```python
from build123d import *

# Parameters (mm, degrees)
F0_R     = 4.5
F1_DEPTH = 3.175
F0_R_2   = 2.25
F2_DEPTH = 1.5875
F3_DEPTH = 13.97
F4_W     = 8.5852
F4_H     = 8.4761770735
F5_DEPTH = 25.4
F6_R     = 3.81


with BuildPart() as f1:
    # F0 (on Top) → F1 (new body)
    with BuildSketch(Plane.XY):
        with BuildLine():
            Line((6.5, -8.5852), (6.5, 0))
            ThreePointArc((6.5, 0), (0, -6.5), (-6.5, 0))
            Line((-6.5, 0), (-6.5, -8.5852))
            Line((-6.5, -8.5852), (6.5, -8.5852))
        make_face()
        with BuildLine():
            ThreePointArc((-6.5, 0), (0, -6.5), (6.5, 0))
            ThreePointArc((6.5, 0), (0, 6.5), (-6.5, 0))
        make_face()
        Circle(F0_R, mode=Mode.SUBTRACT)
    extrude(amount=F1_DEPTH)

    # F0 (on Top) → F2 (join)
    with BuildSketch(Plane.XY):
        Circle(F0_R)
        Circle(F0_R_2, mode=Mode.SUBTRACT)
    extrude(amount=F2_DEPTH)

    # F0 (on Top) → F3 (join)
    with BuildSketch(Plane.XY):
        with BuildLine():
            Line((6.5, -24.3332), (6.5, -8.5852))
            Line((6.5, -8.5852), (-6.5, -8.5852))
            Line((-6.5, -8.5852), (-6.5, -24.3332))
            ThreePointArc((-6.5, -24.3332), (-5.3840768363, -27.0272768363), (-2.69, -28.1432))
            Line((-2.69, -28.1432), (2.69, -28.1432))
            ThreePointArc((2.69, -28.1432), (5.3840768363, -27.0272768363), (6.5, -24.3332))
        make_face()
    extrude(amount=F3_DEPTH)

    # F4 (on face) → F5 (cut)
    with BuildSketch(Plane.YZ.offset(6.5)):
        with BuildLine():
            ThreePointArc((-12.6179837447, 3.175), (-9.7820030962, 4.5000062934), (-8.6270184297, 7.4093770735))
            ThreePointArc((-8.6270184297, 7.4093770735), (-9.8694128853, 10.408782618), (-12.8688184297, 11.6511770735))
            Line((-12.8688184297, 11.6511770735), (-12.8688184297, 3.175))
            Line((-12.8688184297, 3.175), (-12.6179837447, 3.175))
        make_face()
        with BuildLine():
            Line((-12.8688184297, 3.175), (-12.8688184297, 11.6511770735))
            ThreePointArc((-12.8688184297, 11.6511770735), (-17.108762292, 7.2839048265), (-12.6179837447, 3.175))
            Line((-12.6179837447, 3.175), (-12.8688184297, 3.175))
        make_face()
        with Locations((-4.2926, 7.4130885368)):
            Rectangle(F4_W, F4_H)
        with BuildLine():
            ThreePointArc((-12.8688184297, 11.6511770735), (-9.8694128853, 10.408782618), (-8.6270184297, 7.4093770735))
            ThreePointArc((-8.6270184297, 7.4093770735), (-9.7820030962, 4.5000062934), (-12.6179837447, 3.175))
            Line((-12.6179837447, 3.175), (-8.5852, 3.175))
            Line((-8.5852, 3.175), (-8.5852, 11.6511770735))
            Line((-8.5852, 11.6511770735), (-12.8688184297, 11.6511770735))
        make_face()
    extrude(amount=-F5_DEPTH, mode=Mode.SUBTRACT)

    # F6
    f6_edges = [f1.edges().sort_by_distance(p)[0] for p in [
        (6.5, -8.5852, 12.810589),
        (-6.5, -8.5852, 12.810589),
    ]]
    fillet(f6_edges, radius=F6_R)


solid = f1.part
```
The model under review builds one solid part; all positions refer to its coordinate system, in mm. A direction names the side the tool comes from. Give positions to 0.01 mm unless a question says otherwise; leave off trailing zeros. Loops run counter-clockwise (first coordinate to the right, second up) from the corner with the lowest first, then second, coordinate; pieces in that order, holes last. Notation, with made-up numbers: (-24, 67.25) - (-2, 67.25) arc R19 cw to (-2, 88.25) - close; hole circle Ø6 at (26.25, 62.5). An arc over 180 degrees is marked (long way). Answer as a JSON object with one key per item and string values.
Q1. Mouldability with a two-part tool opening along Y and no side actions: class faces 1 (the cylindrical face through (-0.59, 4.46, 2.37)), 2 (the flat face through (0, -8.585, 13)), 3 (the cylindrical face through (5.35, -27.06, 6.89)) as +Y half, -Y half, draft (parallel to the pull), parting line (faces both ways), or undercut.
Worked out:
{"face 1": "undercut", "face 2": "+Y half", "face 3": "-Y half"}
Q2. Add section B-B on y = -9.5. State the section outline as (x, z) points (3 decimals), plus the area to 3 significant figures.
Worked out:
{"outline": "(-6.5, 0) - (6.5, 0) - (6.5, 3.175) - (-6.5, 3.175) - close; (-5.167, 11.651) - (5.167, 11.651) - (5.167, 13.97) - (-5.167, 13.97) - close", "area": "65.2 mm^2"}
Q3. For faces 4 (the flat face through (0, -11, 11.651)), 5 (the cylindrical face through (5.41, -9.73, 12.83)), 6 (the cylindrical face through (-5.41, -9.73, 12.83)), 7 (the flat face through (2, -2, 1.588)), list the 3-axis set-ups (+Z, -Z, +X, -X, +Y, -Y) from which the entire face can be reached by the end or side of a thin tool; tool diameter is ignored.
Worked out:
{"face 4": "+X, -X, +Y", "face 5": "+Z, +X, +Y", "face 6": "+Z, -X, +Y", "face 7": "+Z"}
Q4. Add section C-C on z = 12.25. State the section outline as (x, y) points, plus the area to 3 significant figures.
Worked out:
{"outline": "(-6.5, -24.33) arc R3.81 ccw to (-2.69, -28.14) - (2.69, -28.14) arc R3.81 ccw to (6.5, -24.33) - (6.5, -12.4) arc R3.81 ccw to (2.69, -8.59) - (-2.69, -8.59) arc R3.81 ccw to (-6.5, -12.4) - close", "area": "242 mm^2"}
Q5. To check wall thickness, follow line 1 along Y through (x, z) = (0, 0.75); line 2 along Z through (x, y) = (0.75, -9.5) (3 decimals); line 3 along Y through (x, z) = (-2.25, 12.75). State the ranges of each line that lie inside material, in increasing order.
Worked out:
{"line 1": "y = -28.14 to -2.25, 2.25 to 6.5", "line 2": "z = 0 to 3.175, 11.651 to 13.97", "line 3": "y = -28.14 to -8.59"}
Q6. Add section D-D on y = -3.5. State the section outline as (x, z) points (1 decimal), plus the area to 3 significant figures.
Worked out:
{"outline": "(-6.5, 0) - (6.5, 0) - (6.5, 3.2) - (2.8, 3.2) - (2.8, 1.6) - (-2.8, 1.6) - (-2.8, 3.2) - (-6.5, 3.2) - close", "area": "32.3 mm^2"}
Q7. Insertion check: pin 1 (4 mm diameter, centred on x = -0.5, z = 5.5, fed in from +Y); pin 2 (6 mm diameter, centred on x = 2, y = 0.5, fed in from +Z) (3 decimals); pin 3 (5.5 mm diameter, centred on x = 0, y = 0, fed in from +Z); pin 4 (3.5 mm diameter, centred on x = 0, y = 0, fed in from -Z). Each pin has a flat end and moves straight along its axis. Give the tip position at first contact, or say it passes through.
Worked out:
{"pin 1": "stops at y = -14.51", "pin 2": "stops at z = 3.175", "pin 3": "stops at z = 1.59", "pin 4": "passes through"}
